Autodesk Inventor part; units mm, degrees
ref_plane "YZ Plane" through (0, 0, 0) normal (1, 0, 0) x (0, 1, 0)
ref_plane "XZ Plane" through (0, 0, 0) normal (0, 1, 0) x (-1, 0, 0)
ref_plane "XY Plane" through (0, 0, 0) normal (0, 0, 1) x (1, 0, 0)
sketch "Sketch1" plane through (0, 0, 0) normal (0, 1, 0) x (-1, 0, 0)
  line L0 (5, 15) -> (-5, 15)
  line L1 (-5, 15) -> (-5, -15)
  line L2 (-5, -15) -> (5, -15)
  line L3 (5, -15) -> (5, 15)
  point P0 (0, 0)
  point P1 (5, 0)
  point P2 (0, -15)
  dimension "d0" = 30
  dimension "d1" = 10
extrude "Extrusion1" add sketch "Sketch1" along normal blind 1
sketch "Sketch2" plane through (0, 1, 0) normal (0, 1, 0) x (1, 0, 0)
  line L0 (-5, -15) -> (5, -15)
  point P0 (0, 0)
  point P1 (0, -10)
  dimension "d4" = 5
hole "Hole1" at (0, 1, 10) direction (0, -1, 0) diameter 3.264 depth 4
chamfer "Chamfer1" distance 2 angle 45 1 edges at (5, 0.5, -15)
sketch "Sketch3" plane through (0, 1, 0) normal (0, 1, 0) x (1, 0, 0)
  line L0 (5, -15) -> (5, 13)
  line L1 (3, 15) -> (-5, 15)
  point P0 (0, 0)
  point P1 (2, 12)
  dimension "d15" = 3
  dimension "d16" = 3
hole "Hole2" at (2, 1, -12) direction (0, -1, 0) diameter 2 end through all
properties part number "spring cover" material "Aluminum 6061"
Here's how the part is built. I have some questions about the finished solid (model axes, mm). Coordinates: 2 decimals unless noted, no trailing zeros. Order: outer loops, then holes, each group sorted by start corner. A loop starts at its lowest first (then second) coordinate and runs counter-clockwise, first axis right, second up. Notation, with made-up numbers: M 82.5,39 L 94.5,39 A27 ccw 94.5,57 Z; hole C 77,82.25 d11. An arc over 180 degrees is marked long. Answer as a JSON object with one key per item and string values. Group by question number.
(1) I need wall thicknesses on probe 1 along Z at (x, y) = (0, 0.3); probe 2 along X at (y, z) = (0.7, -12); probe 3 along Z at (x, y) = (2, 0.4). Which ranges of each line are inside material? Lowest first, please.
(2) Suppose I cut it at B-B, the plane z = -12. Please give me the cut outline in (x, y), then the cut area to 3 significant figures.
(3) Suppose I cut it at A-A, the plane x = 2. Please give me the cut outline in (y, z).
(4) Suppose I cut it at C-C, the plane y = 0.5. Please give me the cut outline in (x, z).
(5) If we mould it in two halves opening along X, with no side actions, what happens to faces 1 (the face through (-0.49, 0.493, 11.557)), 2 (the face through (2, 0.5, -13)), 3 (the face through (4, 0.5, -14)), 4 (the face through (-0.1, 0.5, 15))? For each: released by +X, released by -X, zero draft, split by the parting line, or undercut.
Values found:
{
 "1": {"probe 1": "z = -15 to 8.37, 11.63 to 15", "probe 2": "x = -5 to 1, 3 to 5", "probe 3": "z = -15 to -13, -11 to 15"},
 "2": {"outline": "M -5,0 L 1,0 L 1,1 L -5,1 Z; M 3,0 L 5,0 L 5,1 L 3,1 Z", "area": "8.00 mm^2"},
 "3": {"outline": "M 0,-15 L 1,-15 L 1,-13 L 0,-13 Z; M 0,-11 L 1,-11 L 1,15 L 0,15 Z"},
 "4": {"outline": "M -5,-15 L 3,-15 L 5,-13 L 5,15 L -5,15 Z; hole C 0,10 d3.26; hole C 2,-12 d2"},
 "5": {"face 1": "undercut", "face 2": "undercut", "face 3": "released by +X", "face 4": "zero draft"}
}
